Could you check a few things on this model? Use its own coordinates, in mm. Face numbers are marked on the shaded views. A direction names the side the tool comes from. Round coordinates to 2 decimals unless told otherwise and drop trailing zeros. Write each loop counter-clockwise with the first axis right and the second up, starting at its lowest first coordinate (ties: lowest second). Pieces come first, ordered by that corner, then holes. Notation, with made-up numbers: M 88.25,38 L 140.25,38 A20 ccw 140.25,54 Z; hole C -34,-26.75 d3. An arc over 180 degrees is marked long. One line per item, written item: value. Start each with the question number.
(1) If I drill on L1, parallel to Y at x = 13, z = 2.45; L2, parallel to Y at x = 31, z = 0.75; L3, parallel to X at y = 3, z = 3.3, over which ranges is the centre line in solid material (lowest first)?
(2) I want a section at B-B on y = 51. Please give me the cut outline in (x, z), and give its area (3 significant figures).
(3) Which directions (+Z, -Z, +X, -X, +Y, -Y) give clear straight access to the entire face, cutting with the end or side of a thin tool? Please do the marked faces 1, 2, 3, 4 and 5.
(4) I'm going to push flat-ended pins straight in: pin 1 Ø1.5 at (x, z) = (13, 2.5) entering from -Y; pin 2 Ø3 at (y, z) = (4, 2.5) entering from -X; pin 3 Ø1.5 at (y, z) = (52, 1.5) entering from -X. Where does each tip first touch, or does it pass through?
(5) I want a section at A-A on x = 30. Please give me the cut outline in (y, z).
(6) Thinking about a two-plate mould opening in Y: for the marked faces 6, 7 and 8, which applies, released by +Y, released by -Y, zero draft, split by the parting line, or undercut?
(7) I want a section at D-D on x = 19. Please give me the cut outline in (y, z), and give its area (3 significant figures).
(8) I want a section at C-C on y = 17.5. Please give me the cut outline in (x, z), and give its area (3 significant figures).
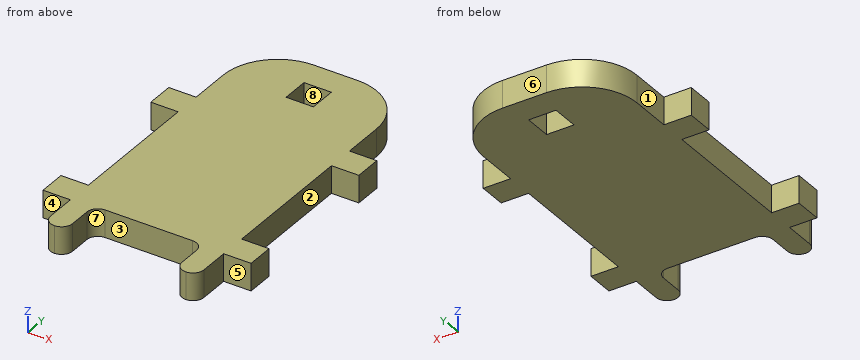
```python
from build123d import *

# Parameters (mm, degrees)
ESQUISSE1_W        = 5
ESQUISSE1_H        = 5
BOSS_EXTRU_1_DEPTH = 5
CONG_1_R           = 2
CONG_2_R           = 2
CONG_3_R           = 10


with BuildPart() as part:
    # Esquisse1 → Boss.-Extru.1 (new body)
    with BuildSketch(Plane.XY):
        Polygon((0, 0), (4, 0), (4, 8), (24, 8), (24, 0), (28, 0), (28, 7.5), (33, 7.5), (33, 12.5), (28, 12.5), (28, 37.5), (33, 37.5), (33, 42.5), (28, 42.5), (28, 60), (0, 60), (0, 42.5), (-5, 42.5), (-5, 37.5), (0, 37.5), (0, 12.5), (-5, 12.5), (-5, 7.5), (0, 7.5), align=None)
        with Locations((14, 52.5)):
            Rectangle(ESQUISSE1_W, ESQUISSE1_H, mode=Mode.SUBTRACT)
    extrude(amount=BOSS_EXTRU_1_DEPTH)

    # Congé1
    cong_1_edges = [part.edges().sort_by_distance(p)[0] for p in [
        (24, 8, 2.5),
        (4, 8, 2.5),
    ]]
    fillet(cong_1_edges, radius=CONG_1_R)

    # Congé2
    cong_2_edges = [part.edges().sort_by_distance(p)[0] for p in [
        (24, 0, 2.5),
        (28, 0, 2.5),
        (0, 0, 2.5),
        (4, 0, 2.5),
    ]]
    fillet(cong_2_edges, radius=CONG_2_R - 0.0001)  # a hair under: the kernel refuses the full size

    # Congé3
    cong_3_edges = [part.edges().sort_by_distance(p)[0] for p in [
        (0, 60, 2.5),
        (28, 60, 2.5),
    ]]
    fillet(cong_3_edges, radius=CONG_3_R)


solid = part.part
```
Found:
1. L1: y = 8 to 50, 55 to 60
1. L2: y = 7.5 to 12.5, 37.5 to 42.5
1. L3: x = 0 to 4, 24 to 28
2. outline: M 0.05,0 L 11.5,0 L 11.5,5 L 0.05,5 Z; M 16.5,0 L 27.95,0 L 27.95,5 L 16.5,5 Z
2. area: 114 mm²
3. face 1: +Z, -Z, -X, +Y
3. face 2: +Z, -Z, +X
3. face 3: +Z, -Z, -Y
3. face 4: +Z, -Z, -X, -Y
3. face 5: +Z, -Z, +X, -Y
4. pin 1: stops at y = 8
4. pin 2: stops at x = 0
4. pin 3: stops at x = 0.08
5. outline: M 7.5,0 L 12.5,0 L 12.5,5 L 7.5,5 Z; M 37.5,0 L 42.5,0 L 42.5,5 L 37.5,5 Z
6. face 6: released by +Y
6. face 7: released by -Y
6. face 8: undercut
7. outline: M 8,0 L 59.95,0 L 59.95,5 L 8,5 Z
7. area: 260 mm²
8. outline: M 0,0 L 28,0 L 28,5 L 0,5 Z
8. area: 140 mm²
